Could you check a few things on this model? Use its own coordinates, in mm. Round coordinates to 2 decimals unless told otherwise and drop trailing zeros. Loops run counter-clockwise (first coordinate to the right, second up) from the corner with the lowest first, then second, coordinate; pieces in that order, holes last. Notation, with made-up numbers: (69.5, 78) -> (76.5, 78) arc R22 cw to (76.5, 104) -> close; hole circle Ø11 at (47, -23). An arc over 180 degrees is marked (long way). Put each result on its own line as item: value. Start each with the question number.
1. I'm going to push flat-ended pins straight in: P1, Ø2, axis at x = -208, z = 6.5, coming from the -Y side; P2, Ø1.5, axis at x = -333.5, z = 8.5, coming from the -Y side; P3, Ø5.5, axis at y = 49, z = 7.5, coming from the -X side; P4, Ø1.5, axis at y = 48.5, z = 7, coming from the +X side. Where does each tip first touch, or does it pass through?
2. Imagine slicing it at B-B, the plane y = 78.5. Please give me the cut outline in (x, z), and give its area (3 significant figures).
3. Imagine slicing it at A-A, the plane z = 6.5. Count the separate pieces of the cut face and the enclosed holes in it, and give its area (3 significant figures).
4. I need wall thicknesses on line 1 (Z direction, x = -301.5, y = 80); line 2 (Y direction, x = -354.5, z = 9); line 3 (Y direction, x = -279, z = 5.5). Which ranges of each line are inside material? Lowest first, please. Write a range as [from, to].
5. Imagine slicing it at C-C, the plane x = -79. Please give me the cut outline in (y, z), and give its area (3 significant figures).
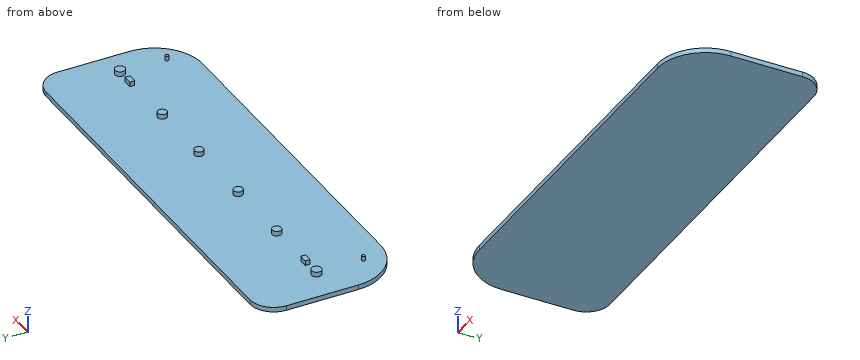
```python
from build123d import *

# Parameters (mm, degrees)
F0_W     = 450
F0_H     = 150
F1_DEPTH = 5
F2_W     = 9
F2_H     = 5
F2_R     = 5.25
F2_R_2   = 4.75
F2_W_2   = 9.5
F2_R_3   = 1.75
F3_DEPTH = 5
F4_R     = 25
F5_R     = 50


with BuildPart() as f1:
    # F0 (on Top) → F1 (new body)
    with BuildSketch(Plane.XY):
        with Locations((-163.935045, 49.38444)):
            Rectangle(F0_W, F0_H)
    extrude(amount=F1_DEPTH)

    # F2 (on face) → F3 (join)
    with BuildSketch(Plane.XY.offset(5)):
        with Locations((-332.185045, 49.38444)):
            Rectangle(F2_W, F2_H)
        with Locations((-353.935045, 49.38444)):
            Circle(F2_R)
        with Locations((-275.935045, 49.38444)):
            Circle(F2_R_2)
        with Locations((-199.935045, 49.38444)):
            Circle(F2_R_2)
        with Locations((-122.935045, 49.38444)):
            Circle(F2_R_2)
        with Locations((-50.935045, 49.38444)):
            Circle(F2_R_2)
        with Locations((32.064955, 49.38444)):
            Circle(F2_R)
        with Locations((12.564955, 49.38444)):
            Rectangle(F2_W_2, F2_H)
        with Locations((-353.935045, 0.38444)):
            Circle(F2_R_3)
        with Locations((32.064955, 0.38444)):
            Circle(F2_R_3)
    extrude(amount=F3_DEPTH)

    # F4
    f4_edges = [f1.edges().sort_by_distance(p)[0] for p in [
        (-388.935045, 124.38444, 2.5),
        (61.064955, 124.38444, 2.5),
    ]]
    fillet(f4_edges, radius=F4_R)

    # F5
    f5_edges = [f1.edges().sort_by_distance(p)[0] for p in [
        (-388.935045, -25.61556, 2.5),
        (61.064955, -25.61556, 2.5),
    ]]
    fillet(f5_edges, radius=F5_R)


solid = f1.part
```
Entries:
1. P1: through
1. P2: y = 46.88
1. P3: x = -388.94
1. P4: x = 37.31
2. outline: (-388.94, 0) -> (61.06, 0) -> (61.06, 5) -> (-388.94, 5) -> close
2. area: 2,250 mm^2
3. separate pieces: 10
3. enclosed holes: 0
3. area: 568 mm^2
4. line 1: [0, 5]
4. line 2: [-1.27, 2.04], [44.16, 54.6]
4. line 3: [45.76, 53.01]
5. outline: (-25.62, 0) -> (124.38, 0) -> (124.38, 5) -> (-25.62, 5) -> close
5. area: 750 mm^2
